Verification items for this drawing (mm, ordinates from the low corner). Give positions to 0.01 mm unless a question says otherwise; leave off trailing zeros. Loops run counter-clockwise (first coordinate to the right, second up) from the corner with the lowest first, then second, coordinate; pieces in that order, holes last. Notation, with made-up numbers: (29, 5) -> (47, 5) arc R13 ccw to (47, 23) -> close; hole circle Ø3 at (14, 79). An arc over 180 degrees is marked (long way). Write each question's results on one line, items separated by ' | '. Start each with the question number.
Item 1: Cross-section at B-B on y = 38.5. Enter the section's corners in (x, z), then the cut area to 3 significant figures.
Item 2: Cross-section at A-A on x = 19. Enter the section's corners in (y, z).
Item 3: Gauge pin test, flat end, axial feed: pin 1 Ø1 at (x, z) = (31.5, 1) entering from -Y. Record the tip position at first contact, or that the pin passes through.
Item 4: Cross-section at C-C on z = 0.3. Enter the section's corners in (x, y).
Item 5: Scan lines: line 1 along Y through (x, z) = (16.5, 1.5); line 2 along X through (y, z) = (40, 0.55). Record each from-to range of solid material in increasing order.
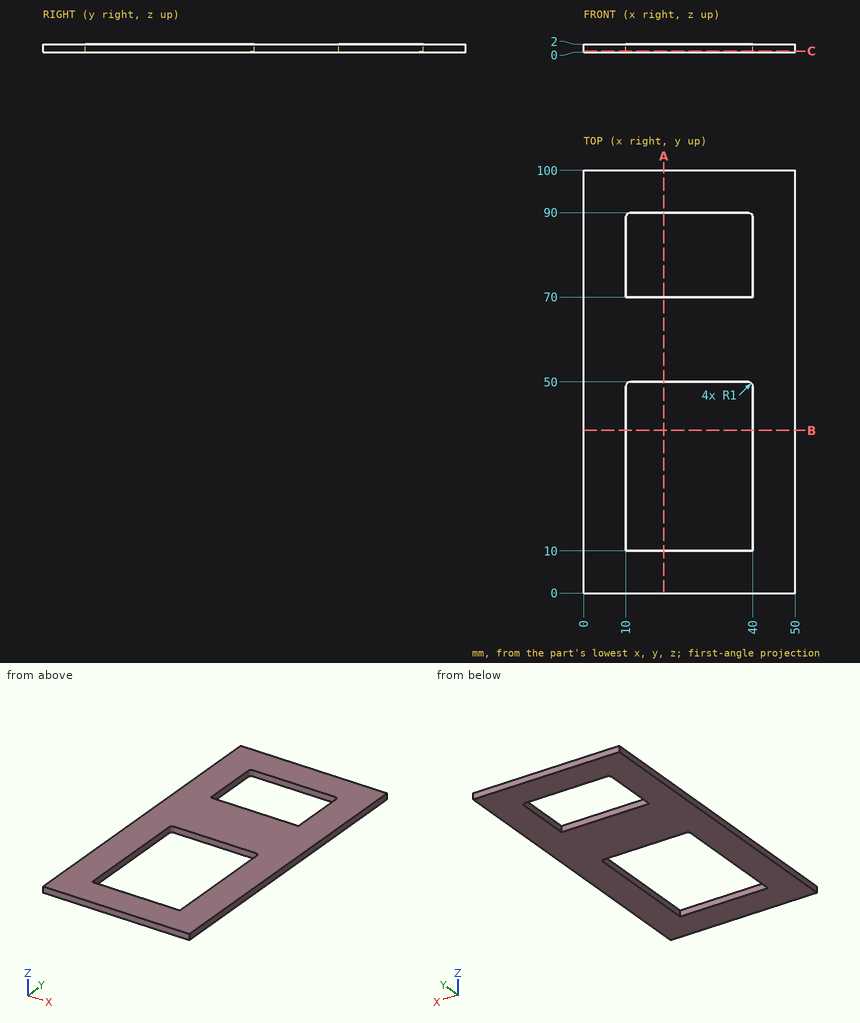
Answer sheet:
1) outline: (0, 0) -> (10, 0) -> (10, 2) -> (0, 2) -> close; (40, 0) -> (50, 0) -> (50, 2) -> (40, 2) -> close | area: 40.0 mm²
2) outline: (0, 0) -> (10, 0) -> (10, 2) -> (0, 2) -> close; (50, 0) -> (70, 0) -> (70, 2) -> (50, 2) -> close; (90, 0) -> (100, 0) -> (100, 2) -> (90, 2) -> close
3) pin 1: stops at y = 0
4) outline: (0, 0) -> (50, 0) -> (50, 100) -> (0, 100) -> close; hole (10, 10) -> (40, 10) -> (40, 49) arc R1 ccw to (39, 50) -> (11, 50) arc R1 ccw to (10, 49) -> close; hole (10, 70) -> (40, 70) -> (40, 89) arc R1 ccw to (39, 90) -> (11, 90) arc R1 ccw to (10, 89) -> close
5) line 1: y = 0 to 10, 50 to 70, 90 to 100 | line 2: x = 0 to 10, 40 to 50
